from build123d import *

# Parameters (mm, degrees)
F1_DEPTH = 1.588
F2_R     = 1.6195
F2_R_2   = 1.5
F3_DEPTH = 1.588


with BuildPart() as f1:
    # F0 (on Top) → F1 (new body)
    with BuildSketch(Plane.XY):
        Polygon((35.56, 11.557), (33.02, 14.097), (33.02, -24.003), (35.56, -21.463), align=None)
        Polygon((33.02, 26.67), (-33.02, 26.67), (-33.02, -26.67), (33.02, -26.67), (33.02, -24.003), (33.02, 14.097), align=None)
    extrude(amount=F1_DEPTH)

    # F2 (on face) → F3 (cut)
    with BuildSketch(Plane.XY.offset(1.588)):
        with Locations((-16.2435, 22.3395)):
            Circle(F2_R)
        with Locations((-17.506, -22.459)):
            Circle(F2_R_2)
        with Locations((31.227971, -17.5895)):
            Circle(F2_R)
        with Locations((31.425, 7.219)):
            Circle(F2_R_2)
    extrude(amount=-F3_DEPTH, mode=Mode.SUBTRACT)


solid = f1.part
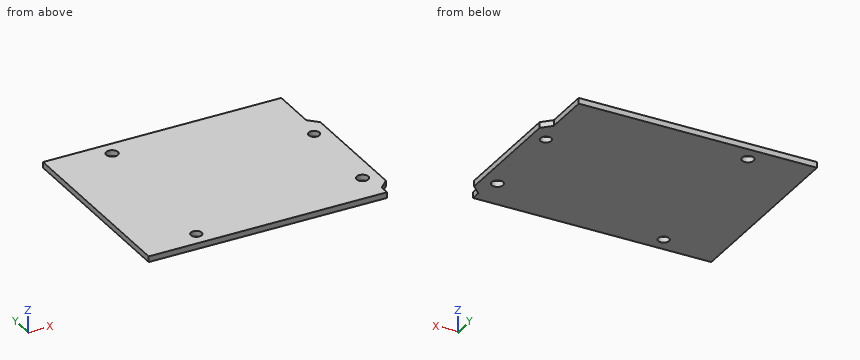
Work out the finished part from the listing and answer in its coordinate system (mm). Coordinates: 2 decimals unless noted, no trailing zeros. Write each loop counter-clockwise with the first axis right and the second up, starting at its lowest first coordinate (ties: lowest second). Pieces come first, ordered by that corner, then holes. Notation, with made-up numbers: M 20.5,6 L 69.5,6 A16 ccw 69.5,21 Z; hole C -32,21.25 d2. An arc over 180 degrees is marked long. Use one line per item in the form item = value. Start each with the question number.
1. The part is cut by section C-C (y = 19.5). Give the vertices of the cut face in (x, z).
2. The part is cut by section A-A (x = 31). Give the vertices of the cut face in (y, z).
3. This flat-tipped pin is pushed along its axis until it touches: P1, Ø0.8, axis at y = -25.5, z = 1, coming from the +X side. Where does it stop, or does it pass through?
4. Straight lines are drawn through the part: probe 1 along X at (y, z) = (-17.5, 1.2) (3 decimals); probe 2 along X at (y, z) = (6, 0.95); probe 3 along Y at (x, z) = (-15.5, 0.5). For each, find the intervals that lie inside material, in ascending order. Write a range as from..to.
5. The part is cut by section B-B (z = 1.3). Give the vertices of the cut face in (x, y) (1 decimal).
Evaluation:
q1.outline = M -33.02,0 L 33.02,0 L 33.02,1.59 L -33.02,1.59 Z
q2.outline = M -26.67,0 L -19.19,0 L -19.19,1.59 L -26.67,1.59 Z; M -15.99,0 L 5.78,0 L 5.78,1.59 L -15.99,1.59 Z; M 8.66,0 L 26.67,0 L 26.67,1.59 L 8.66,1.59 Z
q3.P1 = 33.02
q4.probe_1 = -33.02..29.611, 32.845..35.56
q4.probe_2 = -33.02..30.55, 32.3..35.56
q4.probe_3 = -26.67..20.9, 23.78..26.67
q5.outline = M -33,-26.7 L 33,-26.7 L 33,-24 L 35.6,-21.5 L 35.6,11.6 L 33,14.1 L 33,26.7 L -33,26.7 Z; hole C -17.5,-22.5 d3; hole C -16.2,22.3 d3.2; hole C 31.2,-17.6 d3.2; hole C 31.4,7.2 d3
